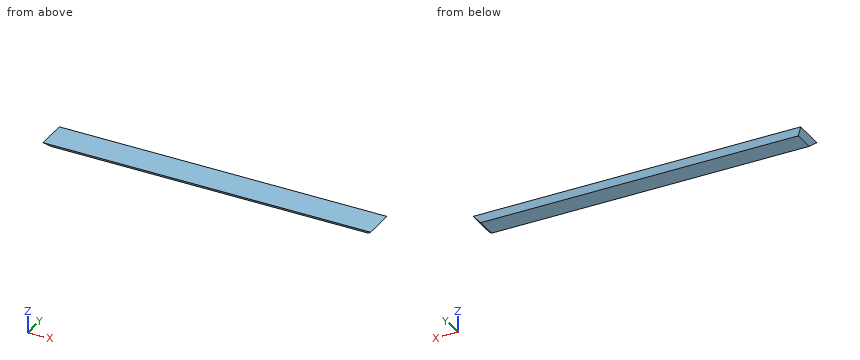
from build123d import *

# Parameters (mm, degrees)
F0_W     = 1600
F0_H     = 150
F1_DEPTH = 12.5
F2_SIZE  = 24.99999


# Not quite as in the source:
# - a fillet or chamfer is up to 0.001 mm smaller than in the source, because OpenCascade refuses the exact size


with BuildPart() as f1:
    # F0 (on Top) → F1 (new body, symmetric)
    with BuildSketch(Plane.XY):
        Rectangle(F0_W, F0_H)
    extrude(amount=F1_DEPTH, both=True)

    # F2 (size 25 in the source; OpenCascade refuses exactly that, so slightly less here)
    f2_edges = [f1.edges().sort_by_distance(p)[0] for p in [
        (0, 75, -12.5),
        (-800, 0, -12.5),
        (0, -75, -12.5),
        (800, 0, -12.5),
    ]]
    chamfer(f2_edges, length=F2_SIZE)


solid = f1.part
Geometry: final body of the model. Coordinates: model frame, mm. Give positions to 0.01 mm unless a question says otherwise; leave off trailing zeros. Write each loop counter-clockwise with the first axis right and the second up, starting at its lowest first coordinate (ties: lowest second). Pieces come first, ordered by that corner, then holes. Notation, with made-up numbers: (62.5, -25) - (66.5, -25) arc R18 ccw to (66.5, -16) - close; hole circle Ø6 at (-24, -11). An arc over 180 degrees is marked (long way). Return JSON: item names as keys, results as strings. Group by question number.
1) First-contact query: P1, Ø2, axis at x = 10.5, z = -2.5, coming from the +Y side; P2, Ø6, axis at y = -25, z = -6.5, coming from the +X side; P3, Ø2, axis at x = -193.5, z = 8.5, coming from the -Y side. Flat tips, straight axial feed; report the tip coordinate or a pass-through.
2) Section C-C on z = 4.5. Return the cut outline in (x, y), plus the area to 3 significant figures.
3) Line query: line 1 (Z direction, x = -238.5, y = -59); line 2 (X direction, y = 60.5, z = 5.25); line 3 (Y direction, x = 172.5, z = -0.75). Output: solid intervals per line, ascending.
Filled in:
{
 "1": {"P1": "stops at y = 61", "P2": "stops at x = 784", "P3": "stops at y = -72"},
 "2": {"outline": "(-792, -67) - (792, -67) - (792, 67) - (-792, 67) - close", "area": "212,000 mm^2"},
 "3": {"line 1": "z = -3.5 to 12.5", "line 2": "x = -792.75 to 792.75", "line 3": "y = -61.75 to 61.75"}
}
